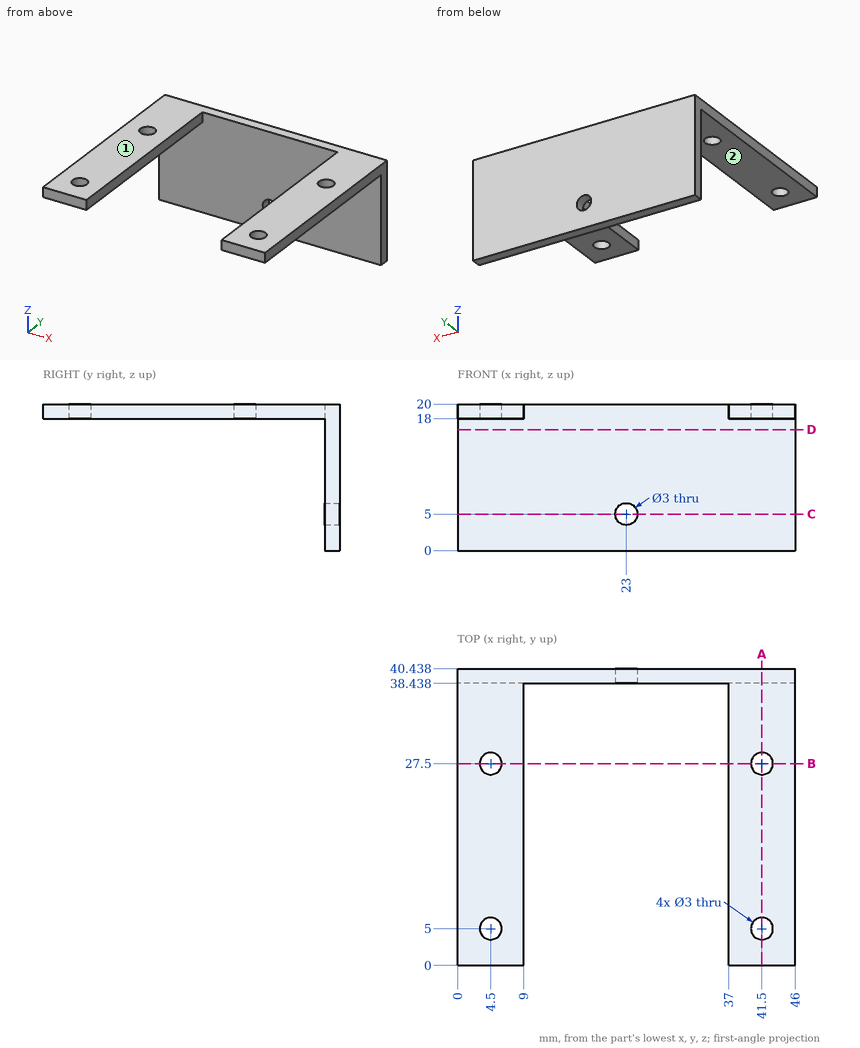
Verification items for this drawing (mm, ordinates from the low corner). A direction names the side the tool comes from. Give positions to 0.01 mm unless a question says otherwise; leave off trailing zeros. Loops run counter-clockwise (first coordinate to the right, second up) from the corner with the lowest first, then second, coordinate; pieces in that order, holes last. Notation, with made-up numbers: M -8,-22 L 12,-22 A21 cw 12,10 Z; hole C 38,-14.5 d5. An arc over 180 degrees is marked long. Answer as a JSON object with one key per item and string values. Group by question number.
Q1. Access from +Z, -Z, +X, -X, +Y, -Y to the whole of each face (thin tool, end or side, straight path). Record for the marked faces 1 and 2.
Q2. Cross-section at C-C on z = 5. Record the cut outline in (x, y).
Q3. Material ranges on line 1 along Y through (x, z) = (41.5, 19.4); line 2 along X through (y, z) = (39.9, 5); line 3 along X through (y, z) = (30.5, 18.75), recorded low to high. Write a range as [from, to].
Q4. Cross-section at D-D on z = 16.5. Record the cut outline in (x, y).
Q5. Go/stop test with flat-tipped pins: P1, Ø2.5, axis at x = 40, y = 18, coming from the -Z side; P2, Ø4, axis at y = 20, z = 14.5, coming from the +X side (3 decimals); P3, Ø12, axis at x = 4.5, y = 5, coming from the +Z side; P4, Ø10, axis at x = 13, z = 5.5, coming from the -Y side. Record where each tip stops, or that it passes through.
Q6. Cross-section at A-A on x = 41.5. Record the cut outline in (y, z), then the cut area to 3 significant figures.
Q7. Cross-section at B-B on y = 27.5. Record the cut outline in (x, z).
Evaluation:
{
 "1": {"face 1": "+Z, +X, -X, +Y, -Y", "face 2": "-Z, +X, -X, -Y"},
 "2": {"outline": "M 0,38.44 L 21.5,38.44 L 21.5,40.44 L 0,40.44 Z; M 24.5,38.44 L 46,38.44 L 46,40.44 L 24.5,40.44 Z"},
 "3": {"line 1": "y = [0, 3.5], [6.5, 26], [29, 40.44]", "line 2": "x = [0, 21.5], [24.5, 46]", "line 3": "x = [0, 9], [37, 46]"},
 "4": {"outline": "M 0,38.44 L 46,38.44 L 46,40.44 L 0,40.44 Z"},
 "5": {"P1": "stops at z = 18", "P2": "passes through", "P3": "stops at z = 20", "P4": "stops at y = 38.44"},
 "6": {"outline": "M 0,18 L 3.5,18 L 3.5,20 L 0,20 Z; M 6.5,18 L 26,18 L 26,20 L 6.5,20 Z; M 29,18 L 38.44,18 L 38.44,0 L 40.44,0 L 40.44,20 L 29,20 Z", "area": "105 mm2"},
 "7": {"outline": "M 0,18 L 3,18 L 3,20 L 0,20 Z; M 6,18 L 9,18 L 9,20 L 6,20 Z; M 37,18 L 40,18 L 40,20 L 37,20 Z; M 43,18 L 46,18 L 46,20 L 43,20 Z"}
}
